Source: CAD feature listing. Evaluate the final solid. Frame: model axes, mm. A direction names the side the tool comes from. Coordinates: 2 decimals unless noted, no trailing zeros. Order: outer loops, then holes, each group sorted by start corner. A loop starts at its lowest first (then second) coordinate and runs counter-clockwise, first axis right, second up. Notation, with made-up numbers: (38.5, 33.5) - (80.5, 33.5) arc R22 ccw to (80.5, 68.5) - close; hole circle Ø1 at (-13, 12). An arc over 180 degrees is marked (long way). One line per question, with ' | ' between items. Start each with the question number.
(1) Section B-B (x = -56.99). Return the cut outline in (y, z), then the cut area to 3 significant figures.
(2) Access query for faces 1 (the flat face through (-53.43, 47, 5)), 2 (the flat face through (-52.25, 19, 5)), 3 (the flat face through (-44.858, 47, 13)), 4 (the flat face through (-60.25, 0, 13)). Directions: +Z, -Z, +X, -X, +Y, -Y. A direction counts if a zero-diameter tool reaches every point of the face in a straight line with its end or side. Return the directions, or none.
(3) Section A-A (y = -30.64). Return the cut outline in (x, z).
(4) Section D-D (y = 14). Return the cut outline in (x, z), then the cut area to 3 significant figures.
(5) Draft query along Y for faces 5 (the flat face through (53.01, 29, 6)), 6 (the flat face through (49, 54, 10.168)), 7 (the flat face through (55, 60.15, 10)). Return one class per face: +Y half, -Y half, draft (parallel to the pull), parting line (faces both ways), or undercut.
(6) Section C-C (z = 13.5). Return the cut outline in (x, y).
(7) Line query: line 1 along Y through (x, z) = (-56.99, 2.5); line 2 along Y through (x, z) = (56.99, 8); line 3 along X through (y, z) = (47, 15.5). Output: solid intervals per line, ascending.
(8) Contact query for flat-ended pins moving along their axis: P1, Ø1.5, axis at x = 14.5, z = 2.5, coming from the +Y side; P2, Ø2.5, axis at x = 56.99, y = -30.64, coming from the -Z side; P3, Ø4, axis at x = -34, y = 19, coming from the +Z side; P4, Ø8, axis at x = -49.02, y = 48.11, coming from the +Z side. Output: stop coordinate, or through.
from build123d import *

# Parameters (mm, degrees)
F0_W     = 123
F0_H     = 70.3
F0_W_2   = 120.5
F0_H_2   = 67.8
F1_DEPTH = 16.5
F0_R     = 1.5
F2_DEPTH = 10.5
F3_W     = 38.5
F3_H     = 7
F4_DEPTH = 9.8
F3_W_2   = 8.5
F3_H_2   = 13.5
F5_DEPTH = 25
F6_W     = 8.3734206855
F6_H     = 6.3322774097
F6_W_2   = 8.5727833211
F7_DEPTH = 25
F9_D     = 5
F11_D    = 5
F13_D    = 5


with BuildPart() as f1:
    # F0 (on Top) → F1 (new body)
    with BuildSketch(Plane.XY):
        Rectangle(F0_W, F0_H)
        Rectangle(F0_W_2, F0_H_2, mode=Mode.SUBTRACT)
    extrude(amount=F1_DEPTH)

    # F0 (on Top) → F2 (join)
    with BuildSketch(Plane.XY):
        Rectangle(F0_W_2, F0_H_2)
        with Locations((-56.99, -6.36)):
            Circle(F0_R, mode=Mode.SUBTRACT)
        with Locations((56.99, -30.64)):
            Circle(F0_R, mode=Mode.SUBTRACT)
        with Locations((-56.99, 30.64)):
            Circle(F0_R, mode=Mode.SUBTRACT)
        with Locations((57.01009, 30.64)):
            Circle(F0_R, mode=Mode.SUBTRACT)
    extrude(amount=F2_DEPTH)

    # F3 (on face) → F4 (cut)
    with BuildSketch(Plane.XY.offset(10.5)):
        with Locations((33.76009, 29.45)):
            Rectangle(F3_W, F3_H)
    extrude(amount=-F4_DEPTH, mode=Mode.SUBTRACT)

    # F3 (on face) → F5 (cut)
    with BuildSketch(Plane.XY.offset(10.5)):
        with Locations((-48, 19.15)):
            Rectangle(F3_W_2, F3_H_2)
    extrude(amount=-F5_DEPTH, mode=Mode.SUBTRACT)

    # F6 (on face) → F7 (join)
    with BuildSketch(Plane(origin=(0, 35.15, 0), x_dir=(-1, 0, 0), z_dir=(0, 1, 0))):
        with Locations((-49.0443054587, 13.3338612951)):
            Rectangle(F6_W, F6_H)
        Polygon((-53.2310158014, 16.5), (-61.5, 16.5), (-61.5, 0), (-53.2310158014, 0), (-53.2310158014, 10.1677225903), align=None)
        with Locations((49.1439905018, 13.3338612951)):
            Rectangle(F6_W_2, F6_H)
        Polygon((53.4303821623, 10.1677225903), (53.4303821623, 0), (61.5, 0), (61.5, 16.5), (53.4303821623, 16.5), align=None)
    extrude(amount=F7_DEPTH)

    # F9 (through all)
    with Locations(Plane(origin=(0, 0, 10.1677225903), x_dir=(1, 0, 0), z_dir=(0, 0, -1))):
        with Locations((-49.0169860423, -48.110447824)):
            Hole(F9_D / 2)

    # F11 (through all)
    with Locations(Plane(origin=(0, 0, 10.1677225903), x_dir=(1, 0, 0), z_dir=(0, 0, -1))):
        with Locations((49.044303596, -47.65)):
            Hole(F11_D / 2)

    # F13 (through all)
    with Locations(Plane.YZ.offset(61.5)):
        with Locations((47.2500026226, 7.9746842384)):
            Hole(F13_D / 2)


solid = f1.part
Response values:
1) outline: (-35.15, 0) - (-7.86, 0) - (-7.86, 10.5) - (-33.9, 10.5) - (-33.9, 16.5) - (-35.15, 16.5) - close; (-4.86, 0) - (29.14, 0) - (29.14, 10.5) - (-4.86, 10.5) - close; (32.14, 0) - (60.15, 0) - (60.15, 16.5) - (33.9, 16.5) - (33.9, 10.5) - (32.14, 10.5) - close; hole circle Ø5 at (47.25, 7.97) | area: 1,080 mm²
2) face 1: -Z, +Y | face 2: +Z, -Z | face 3: +Z, -Z, +Y | face 4: +Z
3) outline: (-61.5, 0) - (55.49, 0) - (55.49, 10.5) - (-60.25, 10.5) - (-60.25, 16.5) - (-61.5, 16.5) - close; (58.49, 0) - (61.5, 0) - (61.5, 16.5) - (60.25, 16.5) - (60.25, 10.5) - (58.49, 10.5) - close
4) outline: (-61.5, 0) - (-52.25, 0) - (-52.25, 10.5) - (-60.25, 10.5) - (-60.25, 16.5) - (-61.5, 16.5) - close; (-43.75, 0) - (61.5, 0) - (61.5, 16.5) - (60.25, 16.5) - (60.25, 10.5) - (-43.75, 10.5) - close | area: 1,220 mm²
5) face 5: undercut | face 6: draft | face 7: +Y half
6) outline: (-61.5, -35.15) - (61.5, -35.15) - (61.5, 60.15) - (44.86, 60.15) - (44.86, 35.15) - (-44.86, 35.15) - (-44.86, 60.15) - (-61.5, 60.15) - close; hole (-60.25, -33.9) - (60.25, -33.9) - (60.25, 33.9) - (-60.25, 33.9) - close; hole circle Ø5 at (-49.02, 48.11); hole circle Ø5 at (49.04, 47.65)
7) line 1: y = -35.15 to -7.86, -4.86 to 29.14, 32.14 to 60.15 | line 2: y = -35.15 to -32.14, -29.14 to 29.14, 32.14 to 44.75, 49.75 to 60.15 | line 3: x = -61.5 to -51.26, -46.78 to -44.86, 44.86 to 46.63, 51.46 to 61.5
8) P1: stops at y = 35.15 | P2: passes through | P3: stops at z = 10.5 | P4: stops at z = 16.5
